from build123d import *

# Parameters (mm, degrees)
SKETCH1_W           = 105
SKETCH1_H           = 150
BOSS_EXTRUDE1_DEPTH = 2
SKETCH2_W           = 105
SKETCH2_H           = 2
BOSS_EXTRUDE2_DEPTH = 130
SKETCH3_R           = 3
CUT_EXTRUDE1_DEPTH  = 10
SKETCH4_R           = 3
CUT_EXTRUDE2_DEPTH  = 10
SKETCH5_R           = 3
CUT_EXTRUDE3_DEPTH  = 10
SKETCH6_R           = 3
CUT_EXTRUDE4_DEPTH  = 10


with BuildPart() as part:
    # Sketch1 → Boss-Extrude1 (new body)
    with BuildSketch(Plane.XY):
        with Locations((52.5, 75)):
            Rectangle(SKETCH1_W, SKETCH1_H)
    extrude(amount=BOSS_EXTRUDE1_DEPTH)

    # Sketch2 → Boss-Extrude2 (add)
    with BuildSketch(Plane(origin=(0, 0, 0), x_dir=(-1, 0, 0), z_dir=(0, 0, -1))):
        with Locations((-52.5, 149)):
            Rectangle(SKETCH2_W, SKETCH2_H)
    extrude(amount=BOSS_EXTRUDE2_DEPTH)

    # Sketch3 → Cut-Extrude1 (cut)
    with BuildSketch(Plane.XY.offset(2)):
        with Locations((15, 30)):
            Circle(SKETCH3_R)
    extrude(amount=-CUT_EXTRUDE1_DEPTH, mode=Mode.SUBTRACT)

    # Sketch4 → Cut-Extrude2 (cut)
    with BuildSketch(Plane.XY.offset(2)):
        with Locations((90, 30)):
            Circle(SKETCH4_R)
    extrude(amount=-CUT_EXTRUDE2_DEPTH, mode=Mode.SUBTRACT)

    # Sketch5 → Cut-Extrude3 (cut)
    with BuildSketch(Plane.XY.offset(2)):
        with Locations((15, 80)):
            Circle(SKETCH5_R)
    extrude(amount=-CUT_EXTRUDE3_DEPTH, mode=Mode.SUBTRACT)

    # Sketch6 → Cut-Extrude4 (cut)
    with BuildSketch(Plane.XY.offset(2)):
        with Locations((90, 80)):
            Circle(SKETCH6_R)
    extrude(amount=-CUT_EXTRUDE4_DEPTH, mode=Mode.SUBTRACT)


solid = part.part
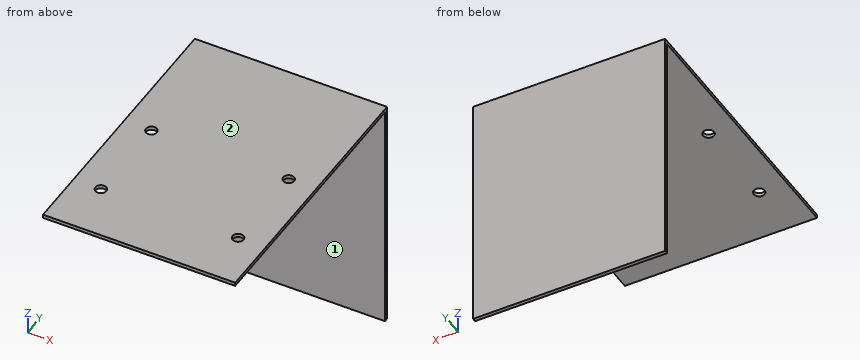
Work out the finished part from the listing and answer in its coordinate system (mm). Face numbers are marked on the shaded views. A direction names the side the tool comes from. Round coordinates to 2 decimals unless told otherwise and drop trailing zeros. Write each loop counter-clockwise with the first axis right and the second up, starting at its lowest first coordinate (ties: lowest second). Pieces come first, ordered by that corner, then holes. Notation, with made-up numbers: (61.25, 12.5) - (73.25, 12.5) arc R15 ccw to (73.25, 25.5) - close; hole circle Ø4 at (12, 38.5). An arc over 180 degrees is marked (long way). Answer in a Markdown table with one row per item. Add a question column.
1. A cutting plane is placed at A-A, the plane y = 80. Determine the outline of the cut face in (x, z).
2. Given pin 1 (6 mm diameter, centred on x = 77.5, z = -33.5, fed in from -Y); pin 2 (1 mm diameter, centred on x = 32.5, y = 18.5, fed in from -Z), each flat-ended and moving along its own axis, determine where each tip first touches the part or whether it passes through.
3. Find the intervals of material crossed by line 1 along Y through (x, z) = (15, 1.45); line 2 along Z through (x, y) = (31.5, 80.5); line 3 along Y through (x, z) = (20, -49.5), in increasing order. Write a range as from..to.
4. A cutting plane is placed at D-D, the plane x = 75.5. Determine the outline of the cut face in (y, z).
5. A cutting plane is placed at C-C, the plane z = -117. Determine the outline of the cut face in (x, y), and give its area (3 significant figures).
6. A cutting plane is placed at B-B, the plane x = 90. Determine the outline of the cut face in (y, z), and give its area (3 significant figures).
7. For the marked faces 1 and 2, determine the directions among +Z, -Z, +X, -X, +Y, -Y from which every point of the face is accessible in a straight line to the end or side of a thin tool.
Worked out:
| question | item | result |
|---|---|---|
| 1 | outline | (0, 0) - (12, 0) - (12, 2) - (0, 2) - close; (18, 0) - (87, 0) - (87, 2) - (18, 2) - close; (93, 0) - (105, 0) - (105, 2) - (93, 2) - close |
| 2 | pin 1 | y = 148 |
| 2 | pin 2 | z = 0 |
| 3 | line 1 | 0..27, 33..77, 83..150 |
| 3 | line 2 | 0..2 |
| 3 | line 3 | 148..150 |
| 4 | outline | (0, 0) - (148, 0) - (148, -130) - (150, -130) - (150, 2) - (0, 2) - close |
| 5 | outline | (0, 148) - (105, 148) - (105, 150) - (0, 150) - close |
| 5 | area | 210 mm^2 |
| 6 | outline | (0, 0) - (27, 0) - (27, 2) - (0, 2) - close; (33, 0) - (77, 0) - (77, 2) - (33, 2) - close; (83, 0) - (148, 0) - (148, -130) - (150, -130) - (150, 2) - (83, 2) - close |
| 6 | area | 536 mm^2 |
| 7 | face 1 | -Z, +X, -X, -Y |
| 7 | face 2 | +Z, +X, -X, +Y, -Y |
